```python
from build123d import *

# Parameters (mm, degrees)
SKETCH_1_R      = 1
SKETCH_1_R_2    = 4
EXTRUDE_1_DEPTH = 1.5


with BuildPart() as part:
    # 草图1 → 凸台-拉伸1 (new body)
    with BuildSketch(Plane.XY):
        with BuildLine():
            Line((-2, -9.082575695), (2, -9.082575695))
            Line((2, -9.082575695), (2, -4.582575695))
            ThreePointArc((2, -4.582575695), (0, 5), (-2, -4.582575695))
            Line((-2, -4.582575695), (-2, -9.082575695))
        make_face()
        with Locations((0, -7.082575695)):
            Circle(SKETCH_1_R, mode=Mode.SUBTRACT)
        Circle(SKETCH_1_R_2, mode=Mode.SUBTRACT)
    extrude(amount=EXTRUDE_1_DEPTH)


solid = part.part
```
The model under review builds one solid part; all positions refer to its coordinate system, in mm. A direction names the side the tool comes from. Coordinates: 2 decimals unless noted, no trailing zeros. Write each loop counter-clockwise with the first axis right and the second up, starting at its lowest first coordinate (ties: lowest second). Pieces come first, ordered by that corner, then holes. Notation, with made-up numbers: (69.25, -35) - (78.25, -35) arc R33 cw to (78.25, 2) - close; hole circle Ø6 at (29.25, 55). An arc over 180 degrees is marked (long way). Answer in a Markdown table with one row per item. Add a question column.
Q1. Consider section D-D on z = 0.3. Give the boundary of the cut face in (x, y), then the cut area to 3 significant figures.
Q2. Consider section A-A on y = 0. Give the boundary of the cut face in (x, z).
Q3. For faces 4 (the face through (2, -4, 1.5)), 5 (the face through (-2, -7, 1)), list the 3-axis set-ups (+Z, -Z, +X, -X, +Y, -Y) from which the entire face can be reached by the end or side of a thin tool; tool diameter is ignored.
Q4. Clearance check with a flat-ended pin moving along its axis: pin 1 (0.8 mm diameter, centred on y = -6.5, z = 0.5, fed in from +X). State where the tip first meets the part, or that it passes through.
Q5. Consider section C-C on x = 3.5. Give the boundary of the cut face in (y, z).
Q6. Draft analysis for pull direction Y (two halves, no side actions). For faces 1 (the face through (2, -7, 1)), 2 (the face through (-0.22, -8.06, 0.74)), 3 (the face through (0, -9.083, 1)), state which applies: +Y half, -Y half, draft (parallel to the pull), parting line (faces both ways), or undercut.
Q7. Consider section B-B on x = 0. Give the boundary of the cut face in (y, z), then the cut area to 3 significant figures.
Q8. To check wall thickness, follow line 1 along Y through (x, z) = (0, 0.95); line 2 along Y through (x, z) = (-0.5, 0.95); line 3 along X through (y, z) = (-2.5, 1.05). State the ranges of each line that lie inside material, in increasing order. Write a range as from..to.
Answers below:
| question | item | result |
|---|---|---|
| 1 | outline | (-2, -9.08) - (2, -9.08) - (2, -4.58) arc R5 ccw (long way) to (-2, -4.58) - close; hole circle Ø8 at (0, 0); hole circle Ø2 at (0, -7.08) |
| 1 | area | 42.0 mm² |
| 2 | outline | (-5, 0) - (-4, 0) - (-4, 1.5) - (-5, 1.5) - close; (4, 0) - (5, 0) - (5, 1.5) - (4, 1.5) - close |
| 3 | face 4 | +Z, +X, -X, +Y, -Y |
| 3 | face 5 | +Z, -Z, -X, -Y |
| 4 | pin 1 | x = 2 |
| 5 | outline | (-3.57, 0) - (-1.94, 0) - (-1.94, 1.5) - (-3.57, 1.5) - close; (1.94, 0) - (3.57, 0) - (3.57, 1.5) - (1.94, 1.5) - close |
| 6 | face 1 | draft |
| 6 | face 2 | undercut |
| 6 | face 3 | -Y half |
| 7 | outline | (-9.08, 0) - (-8.08, 0) - (-8.08, 1.5) - (-9.08, 1.5) - close; (-6.08, 0) - (-4, 0) - (-4, 1.5) - (-6.08, 1.5) - close; (4, 0) - (5, 0) - (5, 1.5) - (4, 1.5) - close |
| 7 | area | 6.12 mm² |
| 8 | line 1 | -9.08..-8.08, -6.08..-4, 4..5 |
| 8 | line 2 | -9.08..-7.95, -6.22..-3.97, 3.97..4.97 |
| 8 | line 3 | -4.33..-3.12, 3.12..4.33 |
